Could you check a few things on this model? Use its own coordinates, in mm. Face numbers are marked on the shaded views. A direction names the side the tool comes from. Give positions to 0.01 mm unless a question says otherwise; leave off trailing zeros. Order: outer loops, then holes, each group sorted by start corner. A loop starts at its lowest first (then second) coordinate and runs counter-clockwise, first axis right, second up.
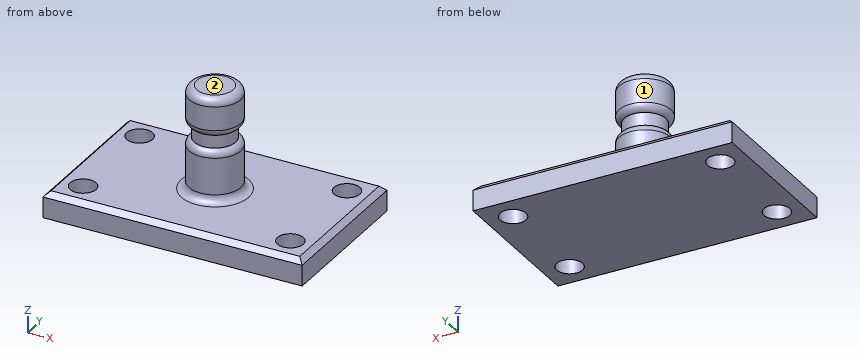
from build123d import *

# Parameters (mm, degrees)
F0_W     = 127
F0_H     = 76.2
F1_DEPTH = 12.7
F2_R     = 6.35
F3_DEPTH = 12.7
F4_W     = 12.7
F4_H     = 50.8
F6_W     = 7.1040334281
F6_H     = 6.35
F9_SIZE  = 2.54


# Not quite as in the source:
# - a fillet or chamfer that OpenCascade refuses, or shapes differently, is made with other operations: its cross-section is extruded or revolved along the edge and cut away or added


with BuildPart() as f1:
    # F0 (on Top) → F1 (new body)
    with BuildSketch(Plane.XY):
        Rectangle(F0_W, F0_H)
    extrude(amount=F1_DEPTH)

    # F2 (on face) → F3 (cut, through all)
    with BuildSketch(Plane.XY.offset(12.7)):
        with Locations((-50.8, 25.4)):
            Circle(F2_R)
        with Locations((-50.8, -25.4)):
            Circle(F2_R)
        with Locations((50.8, -25.4)):
            Circle(F2_R)
        with Locations((50.8, 25.4)):
            Circle(F2_R)
    extrude(amount=-F3_DEPTH, mode=Mode.SUBTRACT)

    # F4 (on Front) → F5 (revolve)
    with BuildSketch(Plane.XZ):
        with Locations((6.35, 38.1)):
            Rectangle(F4_W, F4_H)
    revolve(axis=Axis((0, 0, 38.1), (0, 0, 1)))

    # F6 (on Front) → F7 (revolve, cut)
    with BuildSketch(Plane.XZ):
        with Locations((13.712016714, 41.275)):
            Rectangle(F6_W, F6_H)
    revolve(axis=Axis((0, 0, 12.7), (0, 0, 1)), mode=Mode.SUBTRACT)

    # F8: fillet of radius 3.81 on 4 edges, made by hand

    # F8_s1 → F8_t2 (revolve)
    with BuildSketch(Plane.XZ):
        with BuildLine():
            ThreePointArc((16.51, 12.7), (13.8159231637, 13.8159231637), (12.7, 16.51))
            Line((12.7, 16.51), (12.7, 12.7))
            Line((12.7, 12.7), (16.51, 12.7))
        make_face()
    revolve(axis=Axis((0, 0, 12.7), (0, 0, 1)))

    # F8_s3 → F8_t4 (revolve, cut)
    with BuildSketch(Plane.XZ):
        with BuildLine():
            ThreePointArc((12.7, 34.5078975516), (12.0008519733, 36.7076020772), (10.16, 38.1))
            Line((10.16, 38.1), (12.7, 38.1))
            Line((12.7, 38.1), (12.7, 34.5078975516))
        make_face()
    revolve(axis=Axis((0, 0, 38.1), (0, 0, 1)), mode=Mode.SUBTRACT)

    # F8_s5 → F8_t6 (revolve, cut)
    with BuildSketch(Plane.XZ):
        with BuildLine():
            ThreePointArc((10.16, 44.45), (12.0008519733, 45.8423979228), (12.7, 48.0421024484))
            Line((12.7, 48.0421024484), (12.7, 44.45))
            Line((12.7, 44.45), (10.16, 44.45))
        make_face()
    revolve(axis=Axis((0, 0, 44.45), (0, 0, 1)), mode=Mode.SUBTRACT)

    # F8_s7 → F8_t8 (revolve, cut)
    with BuildSketch(Plane.XZ):
        with BuildLine():
            ThreePointArc((12.7, 59.69), (11.5840768363, 62.3840768363), (8.89, 63.5))
            Line((8.89, 63.5), (12.7, 63.5))
            Line((12.7, 63.5), (12.7, 59.69))
        make_face()
    revolve(axis=Axis((0, 0, 63.5), (0, 0, 1)), mode=Mode.SUBTRACT)

    # F9
    f9_edges = [f1.edges().sort_by_distance(p)[0] for p in [
        (0, -38.1, 12.7),
        (-63.5, 0, 12.7),
        (63.5, 0, 12.7),
        (0, 38.1, 12.7),
    ]]
    chamfer(f9_edges, length=F9_SIZE)


solid = f1.part
Item 1: Imagine slicing it at C-C on y = 0. List the corners of the cut face in (x, z) for me.
Findings:
outline: (-63.5, 0) - (63.5, 0) - (63.5, 10.16) - (60.96, 12.7) - (16.51, 12.7) arc R3.81 cw to (12.7, 16.51) - (12.7, 34.51) arc R3.81 ccw to (10.16, 38.1) - (10.16, 44.45) arc R3.81 ccw to (12.7, 48.04) - (12.7, 59.69) arc R3.81 ccw to (8.89, 63.5) - (-8.89, 63.5) arc R3.81 ccw to (-12.7, 59.69) - (-12.7, 48.04) arc R3.81 ccw to (-10.16, 44.45) - (-10.16, 38.1) arc R3.81 ccw to (-12.7, 34.51) - (-12.7, 16.51) arc R3.81 cw to (-16.51, 12.7) - (-60.96, 12.7) - (-63.5, 10.16) - close
Item 2: Imagine slicing it at B-B on y = 25.4. List the corners of the cut face in (x, z) for me.
Findings:
outline: (-63.5, 0) - (-57.15, 0) - (-57.15, 12.7) - (-60.96, 12.7) - (-63.5, 10.16) - close; (-44.45, 0) - (44.45, 0) - (44.45, 12.7) - (-44.45, 12.7) - close; (57.15, 0) - (63.5, 0) - (63.5, 10.16) - (60.96, 12.7) - (57.15, 12.7) - close
Item 3: Imagine slicing it at D-D on x = 0. List the corners of the cut face in (y, z) for me.
Findings:
outline: (-38.1, 0) - (38.1, 0) - (38.1, 10.16) - (35.56, 12.7) - (16.51, 12.7) arc R3.81 cw to (12.7, 16.51) - (12.7, 34.51) arc R3.81 ccw to (10.16, 38.1) - (10.16, 44.45) arc R3.81 ccw to (12.7, 48.04) - (12.7, 59.69) arc R3.81 ccw to (8.89, 63.5) - (-8.89, 63.5) arc R3.81 ccw to (-12.7, 59.69) - (-12.7, 48.04) arc R3.81 ccw to (-10.16, 44.45) - (-10.16, 38.1) arc R3.81 ccw to (-12.7, 34.51) - (-12.7, 16.51) arc R3.81 cw to (-16.51, 12.7) - (-35.56, 12.7) - (-38.1, 10.16) - close
Item 4: Please list where these lines run through material, in increasing order: line 1 along X through (y, z) = (-25, 7); line 2 along Y through (x, z) = (-50.8, 5); line 3 along Z through (x, y) = (-37, -21.5).
Findings:
line 1: x = -63.5 to -57.14, -44.46 to 44.46, 57.14 to 63.5
line 2: y = -38.1 to -31.75, -19.05 to 19.05, 31.75 to 38.1
line 3: z = 0 to 12.7
Item 5: Imagine slicing it at A-A on x = -50.8. List the corners of the cut face in (y, z) for me.
Findings:
outline: (-38.1, 0) - (-31.75, 0) - (-31.75, 12.7) - (-35.56, 12.7) - (-38.1, 10.16) - close; (-19.05, 0) - (19.05, 0) - (19.05, 12.7) - (-19.05, 12.7) - close; (31.75, 0) - (38.1, 0) - (38.1, 10.16) - (35.56, 12.7) - (31.75, 12.7) - close
Item 6: For pin 1 (1 mm diameter, centred on x = 37.5, y = 11.5, fed in from +Z); pin 2 (6 mm diameter, centred on y = 1, z = 32.5, fed in from +X), each with a flat end and sliding along its axis, tell me the tip position at first contact or that it passes through.
Findings:
pin 1: stops at z = 12.7
pin 2: stops at x = 12.7
Item 7: For the marked faces 1 and 2, which set-ups out of +Z, -Z, +X, -X, +Y, -Y let a thin tool reach every point of the face, with its end or its side?
Findings:
face 1: +Z
face 2: +Z, +X, -X, +Y, -Y
